Input: part model. Units: mm. Frame: model coordinates. A direction names the side the tool comes from. Round coordinates to 2 decimals unless told otherwise and drop trailing zeros. Loops run counter-clockwise (first coordinate to the right, second up) from the corner with the lowest first, then second, coordinate; pieces in that order, holes last.
1) First-contact query: pin 1 (2 mm diameter, centred on x = -11.5, z = 7.5, fed in from +Y); pin 2 (1 mm diameter, centred on y = 0, z = 1.5, fed in from -X); pin 3 (1.5 mm diameter, centred on x = -14.5, y = -5.5, fed in from -Z); pin 4 (17.5 mm diameter, centred on x = -4, z = -40.5, fed in from +Y). Flat tips, straight axial feed; report the tip coordinate or a pass-through.
2) Ray query, line 1 along Z through (x, y) = (-18.5, 5.75); line 2 along Z through (x, y) = (-33, 7); line 3 along Y through (x, z) = (15, -12.5). Return the intervals inside material, ascending.
3) Section D-D, the plane y = -3.5. Return loops of the section in (x, z), and give its area (3 significant figures).
4) Access query for faces 4 (the face through (-9, 3, -35)), 5 (the face through (-10, 1, 20.835)), 6 (the face through (-10, 9.251, 19)), 7 (the face through (-9, 0, -10)), 8 (the face through (56.071, 1, 19)). Directions: +Z, -Z, +X, -X, +Y, -Y. A direction counts if a zero-diameter tool reaches every point of the face in a straight line with its end or side. Return the directions, or none.
5) Section A-A, the plane y = 6.5. Return loops of the section in (x, z), and give its area (3 significant figures).
6) Draft query along X for faces 1 (the face through (-9, 3, -10)), 2 (the face through (-10.36, 6.45, -45.91)), 3 (the face through (-8.655, 1.479, -52.902)). Return one class per face: pulls with the +X half, pulls with the -X half, needs draft (parallel to the pull), parting line crosses it, or undercut.
7) Section B-B, the plane z = -32. Return loops of the section in (x, y).
8) Section C-C, the plane x = 25. Return loops of the section in (y, z), and give its area (3 significant figures).
from build123d import *

# Parameters (mm, degrees)
BOSS_EXTRUDE1_DEPTH = 3
SKETCH2_R           = 14
SKETCH2_R_2         = 11
BOSS_EXTRUDE2_DEPTH = 7
SKETCH3_W           = 130
SKETCH3_H           = 17
BOSS_EXTRUDE3_DEPTH = 3


with BuildPart() as part:
    # Sketch1 → Boss-Extrude1 (new body)
    with BuildSketch(Plane(origin=(0, 0, 0), x_dir=(1, 0, 0), z_dir=(0, 1, 0))):
        with BuildLine():
            Line((-48.929144451, -17.835062273), (31.070855549, -17.835062273))
            Line((31.070855549, -17.835062273), (6.985518971, 43.196988966))
            ThreePointArc((6.985518971, 43.196988966), (-8.929144451, 52.904273338), (-24.843807874, 43.196988966))
            Line((-24.843807874, 43.196988966), (-48.929144451, -17.835062273))
        make_face()
    extrude(amount=BOSS_EXTRUDE1_DEPTH)

    # Sketch2 → Boss-Extrude2 (add)
    with BuildSketch(Plane(origin=(0, 3, 0), x_dir=(1, 0, 0), z_dir=(0, 1, 0))):
        with Locations((-8.929144451, 35.004937727)):
            Circle(SKETCH2_R)
        with Locations((-8.929144451, 35.004937727)):
            Circle(SKETCH2_R_2, mode=Mode.SUBTRACT)
    extrude(amount=BOSS_EXTRUDE2_DEPTH)

    # Sketch3 → Boss-Extrude3 (add)
    with BuildSketch(Plane.XY.offset(17.835062273)):
        with Locations((-8.929144451, 0.75050315)):
            Rectangle(SKETCH3_W, SKETCH3_H)
    extrude(amount=BOSS_EXTRUDE3_DEPTH)


solid = part.part
Final values:
1. pin 1: stops at y = 3
1. pin 2: stops at x = -42.68
1. pin 3: stops at z = 17.84
1. pin 4: stops at y = 10
2. line 1: z = -45.22 to -40.43, -29.58 to -24.79, 17.84 to 20.84
2. line 2: z = 17.84 to 20.84
2. line 3: y = 0 to 3
3. outline: (-73.93, 17.84) - (56.07, 17.84) - (56.07, 20.84) - (-73.93, 20.84) - close
3. area: 390 mm2
4. face 4: +Y
4. face 5: +Z, +X, -X, +Y, -Y
4. face 6: +Z, +X, -X, +Y
4. face 7: -Z, +X, -X, -Y
4. face 8: +Z, -Z, +X, +Y, -Y
5. outline: (-73.93, 17.84) - (56.07, 17.84) - (56.07, 20.84) - (-73.93, 20.84) - close; circle Ø28 at (-8.93, -35); hole circle Ø22 at (-8.93, -35)
5. area: 626 mm2
6. face 1: needs draft
6. face 2: undercut
6. face 3: parting line crosses it
7. outline: (-29.26, 0) - (11.4, 0) - (11.4, 3) - (4.74, 3) - (4.74, 10) - (1.65, 10) - (1.65, 3) - (-19.51, 3) - (-19.51, 10) - (-22.6, 10) - (-22.6, 3) - (-29.26, 3) - close
8. outline: (-7.75, 17.84) - (0, 17.84) - (0, 2.45) - (3, 2.45) - (3, 17.84) - (9.25, 17.84) - (9.25, 20.84) - (-7.75, 20.84) - close
8. area: 97.2 mm2
